```python
from build123d import *

# Parameters (mm, degrees)
SKETCH_W     = 33.55
SKETCH_H     = 51.75
PAD_DEPTH    = 1.73
SKETCH001_W  = 29.2
SKETCH001_H  = 43
POCKET_DEPTH = 5
CHAMFER_SIZE = 1


with BuildPart() as part:
    # Sketch → Pad (new body)
    with BuildSketch(Plane.XY):
        Rectangle(SKETCH_W, SKETCH_H)
    extrude(amount=PAD_DEPTH)

    # Sketch001 (on Face6 of Pad) → Pocket (cut)
    with BuildSketch(Plane.XY.offset(1.73)):
        with Locations((0, 1.125)):
            Rectangle(SKETCH001_W, SKETCH001_H)
    extrude(amount=-POCKET_DEPTH, mode=Mode.SUBTRACT)

    # Chamfer
    chamfer_edges = [part.edges().sort_by_distance(p)[0] for p in [
        (0, -20.375, 1.73),
    ]]
    chamfer(chamfer_edges, length=CHAMFER_SIZE)


solid = part.part
```
Verification items for the finished model (mm, model axes). A direction names the side the tool comes from. Give positions to 0.01 mm unless a question says otherwise; leave off trailing zeros. Write each loop counter-clockwise with the first axis right and the second up, starting at its lowest first coordinate (ties: lowest second). Pieces come first, ordered by that corner, then holes. Notation, with made-up numbers: (60.5, 79) - (105.5, 79) arc R28 ccw to (105.5, 104) - close; hole circle Ø3 at (9.25, 11). An arc over 180 degrees is marked (long way). Put each result on its own line as item: value.
Q1. Scan lines: probe 1 along X at (y, z) = (-11, 0.4) (3 decimals); probe 2 along Y at (x, z) = (0.5, 0.2) (3 decimals); probe 3 along Y at (x, z) = (-3, 1.3) (3 decimals). Record each from-to range of solid material in increasing order. Write a range as from..to.
Result:
probe 1: -16.775..-14.6, 14.6..16.775
probe 2: -25.875..-20.375, 22.625..25.875
probe 3: -25.875..-20.945, 22.625..25.875
Q2. Mould release check, pull along X, two halves, no side actions. Record for faces 3 (the face through (-16.775, 0, 1)), 4 (the face through (0, -25.875, 1)), 5 (the face through (0, 22.625, 1)): released by +X, released by -X, zero draft, split by the parting line, or undercut.
Result:
face 3: released by -X
face 4: zero draft
face 5: undercut
Q3. Section check C-C on z = 0.35. Record the cut outline in (x, y) (3 decimals).
Result:
outline: (-16.775, -25.875) - (16.775, -25.875) - (16.775, 25.875) - (-16.775, 25.875) - close; hole (-14.6, -20.375) - (14.6, -20.375) - (14.6, 22.625) - (-14.6, 22.625) - close
Q4. Set-up check for faces 1 (the face through (-0.204, -20.868, 1.223)), 2 (the face through (15, 0, 0)): record each of +Z, -Z, +X, -X, +Y, -Y from which the full face is reachable in a straight line by a thin tool's end or side.
Result:
face 1: +Z
face 2: -Z, +X, -X, +Y, -Y
Q5. Section check B-B on x = 7.5. Record the cut outline in (y, z) (3 decimals).
Result:
outline: (-25.875, 0) - (-20.375, 0) - (-20.375, 0.73) - (-21.375, 1.73) - (-25.875, 1.73) - close; (22.625, 0) - (25.875, 0) - (25.875, 1.73) - (22.625, 1.73) - close
Q6. Section check A-A on y = 5. Record the cut outline in (x, z) (3 decimals), and give its area (3 significant figures).
Result:
outline: (-16.775, 0) - (-14.6, 0) - (-14.6, 1.73) - (-16.775, 1.73) - close; (14.6, 0) - (16.775, 0) - (16.775, 1.73) - (14.6, 1.73) - close
area: 7.53 mm2
